Input: dimensioned drawing with shaded views. Units: mm. Origin: part minimum x, y, z. Round coordinates to 2 decimals unless told otherwise and drop trailing zeros. Loops run counter-clockwise (first coordinate to the right, second up) from the corner with the lowest first, then second, coordinate; pieces in that order, holes last.
1) Ray query, line 1 along Z through (x, y) = (2, 1.75); line 2 along Z through (x, y) = (19.5, 2.05); line 3 along X through (y, z) = (2.35, 13.25). Return the intervals inside material, ascending.
2) First-contact query: pin 1 (1.5 mm diameter, centred on x = 11.5, y = 1, fed in from -Z); pin 2 (0.9 mm diameter, centred on x = 11.5, y = 2, fed in from +Z); pin 3 (1.5 mm diameter, centred on y = 1, z = 1, fed in from -X). Flat tips, straight axial feed; report the tip coordinate or a pass-through.
3) Section A-A, the plane z = 7.25. Return loops of the section in (x, y), and give its area (3 significant figures).
4) Section B-B, the plane x = 19.5. Return loops of the section in (y, z), and give its area (3 significant figures).
5) Section D-D, the plane z = 23.5. Return loops of the section in (x, y), and give its area (3 significant figures).
6) Section C-C, the plane z = 1.75. Return loops of the section in (x, y).
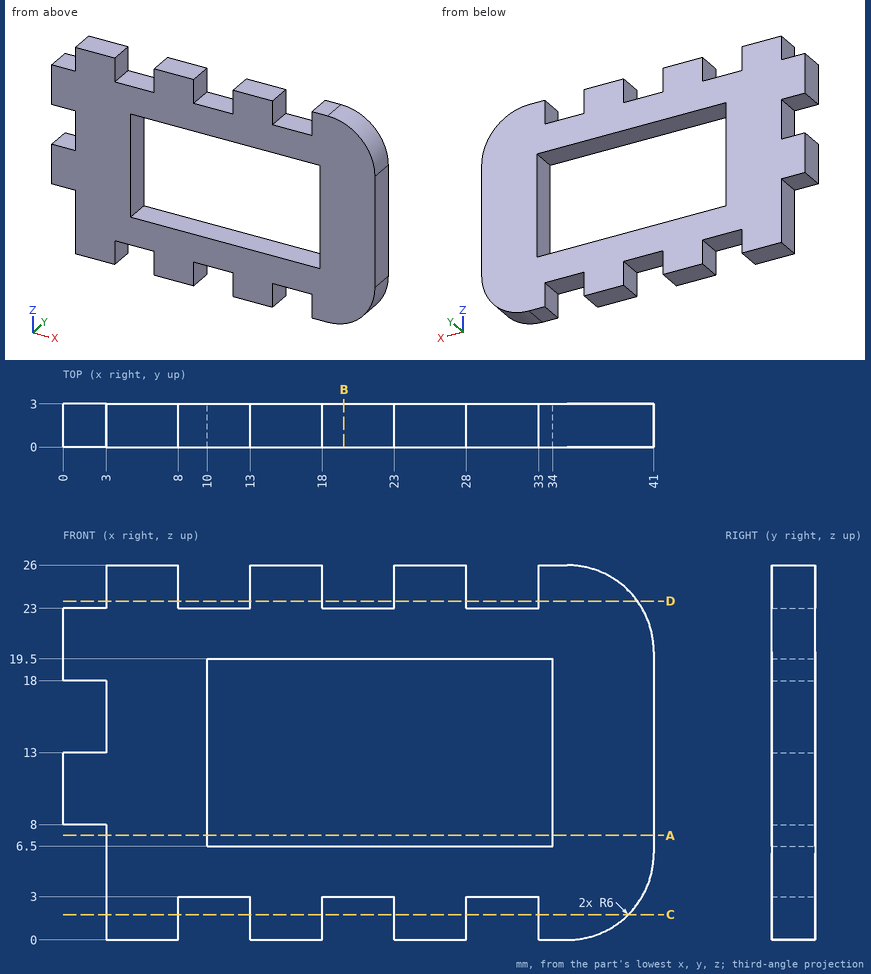
Final values:
1. line 1: z = 8 to 13, 18 to 23
1. line 2: z = 3 to 6.5, 19.5 to 23
1. line 3: x = 3 to 10, 34 to 41
2. pin 1: stops at z = 3
2. pin 2: stops at z = 23
2. pin 3: stops at x = 3
3. outline: (3, 0) - (10, 0) - (10, 3) - (3, 3) - close; (34, 0) - (41, 0) - (41, 3) - (34, 3) - close
3. area: 42.0 mm2
4. outline: (0, 3) - (3, 3) - (3, 6.5) - (0, 6.5) - close; (0, 19.5) - (3, 19.5) - (3, 23) - (0, 23) - close
4. area: 21.0 mm2
5. outline: (3, 0) - (8, 0) - (8, 3) - (3, 3) - close; (13, 0) - (18, 0) - (18, 3) - (13, 3) - close; (23, 0) - (28, 0) - (28, 3) - (23, 3) - close; (33, 0) - (39.87, 0) - (39.87, 3) - (33, 3) - close
5. area: 65.6 mm2
6. outline: (3, 0) - (8, 0) - (8, 3) - (3, 3) - close; (13, 0) - (18, 0) - (18, 3) - (13, 3) - close; (23, 0) - (28, 0) - (28, 3) - (23, 3) - close; (33, 0) - (39.24, 0) - (39.24, 3) - (33, 3) - close
